from build123d import *

# Parameters (mm, degrees)
F0_W     = 440
F0_H     = 500
F1_DEPTH = 20
F2_W     = 190
F2_H     = 40
F3_DEPTH = 20
F4_R     = 30
F6_D     = 5


# Not quite as in the source:
# - a feature names something its author has since deleted; it is built from what else it names


with BuildPart() as f1:
    # F0 (on Right) → F1 (new body)
    with BuildSketch(Plane.YZ):
        with Locations((31.3553263247, 6.565798074)):
            Rectangle(F0_W, F0_H)
    extrude(amount=F1_DEPTH)

    # F2 (on face) → F3 (cut, through all)
    with BuildSketch(Plane.YZ.offset(20)):
        with Locations((-63.6446736753, -223.434201926)):
            Rectangle(F2_W, F2_H)
        with Locations((126.3553263247, -223.434201926)):
            Rectangle(F2_W, F2_H)
    extrude(amount=-F3_DEPTH, mode=Mode.SUBTRACT)

    # F4
    f4_edges = [f1.edges().sort_by_distance(p)[0] for p in [
        (10, -158.644674, -203.434202),
        (10, 221.355326, -203.434202),
    ]]
    fillet(f4_edges, radius=F4_R)

    # F6 (through all)
    with Locations(Plane(origin=(0, 0, 0), x_dir=(0, -1, 0), z_dir=(-1, 0, 0))):
        with Locations((148.6446736753, -183.434201926), (58.6446736753, -183.434201926), (-31.3553263247, -183.434201926), (-121.3553263247, -183.434201926), (-211.3553263247, -183.434201926), (148.6446736753, 136.565798074), (58.6446736753, 136.565798074), (-31.3553263247, 136.565798074), (-121.3553263247, 136.565798074), (-211.3553263247, 136.565798074)):
            Hole(F6_D / 2)


solid = f1.part
Check sheet for the modelled part. Datum: model origin and axes. Units: mm. A direction names the side the tool comes from. Give positions to 0.01 mm unless a question says otherwise; leave off trailing zeros. Loops run counter-clockwise (first coordinate to the right, second up) from the corner with the lowest first, then second, coordinate; pieces in that order, holes last. Notation, with made-up numbers: M 31.5,26 L 60.5,26 A9 cw 60.5,33 Z; hole C 7.5,82 d2. An arc over 180 degrees is marked long. Answer as a JSON object with one key per item and string values. Group by question number.
Q1. Cross-section at A-A on x = 11.25. Give the number of separate pieces and of enclosed holes in the cut face, then the cut area to 3 significant figures.
Q2. Cross-section at B-B on y = -107.5. Record the cut outline in (x, z), then the cut area to 3 significant figures.
Q3. Access from +Z, -Z, +X, -X, +Y, -Y to the whole of each face (thin tool, end or side, straight path). Record for faces 5 (the flat face through (10, 236, -243.434)), 6 (the flat face through (10, -158.645, -239)).
Q4. Material ranges on line 1 along Y through (x, z) = (18, 137.5); line 2 along Z through (x, y) = (12.25, 210.5); line 3 along Z through (x, y) = (15.25, 21), recorded low to high. Write a range as [from, to].
Q5. Go/stop test with a flat-tipped pin: P1, Ø6, axis at x = 7, y = 89.5, coming from the -Z side. Record where the tip stops, or that it passes through.
Q6. Release check for a two-part mould opening along Y. For faces 1 (the cylindrical face through (9.86, -150.09, -212.456)), 2 (the flat face through (10, 28, 256.566)), 3 (the flat face through (10, 251.355, 3)), 4 (the flat face through (10, 34, -203.434)) record: released by +Y, released by -Y, zero draft, split by the parting line, or undercut.
Evaluation:
{
 "1": {"separate pieces": "1", "enclosed holes": "10", "area": "205,000 mm2"},
 "2": {"outline": "M 0,-203.43 L 20,-203.43 L 20,256.57 L 0,256.57 Z", "area": "9,200 mm2"},
 "3": {"face 5": "-Z, +X, -X, +Y, -Y", "face 6": "-Z, +X, -X"},
 "4": {"line 1": "y = [-188.64, -150.96], [-146.33, -60.96], [-56.33, 29.04], [33.67, 119.04], [123.67, 209.04], [213.67, 251.36]", "line 2": "z = [-210.34, -185.78], [-181.09, 134.22], [138.91, 256.57]", "line 3": "z = [-203.43, 256.57]"},
 "5": {"P1": "stops at z = -203.43"},
 "6": {"face 1": "undercut", "face 2": "zero draft", "face 3": "released by +Y", "face 4": "undercut"}
}
